Autodesk Inventor part; units mm, degrees
ref_plane "YZ Plane" through (0, 0, 0) normal (1, 0, 0) x (0, 1, 0)
ref_plane "XZ Plane" through (0, 0, 0) normal (0, 1, 0) x (-1, 0, 0)
ref_plane "XY Plane" through (0, 0, 0) normal (0, 0, 1) x (1, 0, 0)
sketch "Sketch1" plane through (0, 0, 0) normal (1, 0, 0) x (0, 1, 0)
  arc A0 (6.25, -17.1964) -> (-6.25, -17.1964) centre (0, -20) ccw
  line L0 (-6.25, -17.1964) -> (-6.25, -42.8036)
  line L1 (-6.25, -30) -> (6.25, -30) construction
  line L2 (0, 0) -> (0, -137.3205) construction
  arc A1 (-6.25, -42.8036) -> (6.25, -42.8036) centre (0, -40) ccw
  circle A2 centre (0, 0) radius 40 construction
  circle A3 centre (0, -20) radius 20 construction
  line L3 (6.25, -17.1964) -> (6.25, -42.8036)
  line L4 (0, 0) -> (17.3205, -10) construction
  line L5 (17.3205, -10) -> (34.641, -20) construction
  line L6 (-25, -137.3205) -> (25, -137.3205) construction
  line L7 (-18, -125.3205) -> (-18, -29)
  line L8 (22.5, -125.3205) -> (22.5, -100.3205)
  line L9 (-25, -120) -> (25, -120) construction
  line L10 (25, -120) -> (25, -137.3205) construction
  line L11 (-25, -120) -> (-25, -137.3205) construction
  line L12 (22.5, -109.2705) -> (17.5, -109.2705)
  line L13 (17.5, -109.2705) -> (17.5, -117.3705)
  line L14 (17.5, -117.3705) -> (22.5, -117.3705)
  line L15 (-15, -106.3205) -> (17.5, -106.3205) construction
  line L16 (17.5, -106.3205) -> (17.5, -149.3205) construction
  line L17 (17.5, -149.3205) -> (-15, -149.3205) construction
  line L18 (-15, -149.3205) -> (-15, -106.3205) construction
  line L19 (-15, -106.3205) -> (17.5, -149.3205) construction
  line L20 (17.5, -106.3205) -> (-15, -149.3205) construction
  line L21 (1.25, -106.3205) -> (1.25, -149.3205) construction
  line L22 (22.5, -109.3205) -> (17.5, -109.3205) construction
  line L23 (17.5, -117.3205) -> (22.5, -117.3205) construction
  line L24 (17.5, -113.3205) -> (22.5, -113.3205) construction
  line L25 (-18, -100.3205) -> (22.5, -100.3205) construction
  circle A4 centre (0, 0) radius 4 construction
  circle A5 centre (20, -103.3205) radius 1.75 construction
  line L26 (20, -103.3205) -> (20, -123.3205) construction
  circle A6 centre (20, -123.3205) radius 1.75 construction
  line L27 (-18, -109.2705) -> (-13, -109.2705)
  line L28 (-13, -109.2705) -> (-13, -117.3705)
  line L29 (-13, -117.3705) -> (-18, -117.3705)
  line L30 (-15.5, -103.3205) -> (-15.5, -123.3205) construction
  line L31 (-15.5, -103.3205) -> (20, -103.3205) construction
  line L32 (-15.5, -123.3205) -> (20, -123.3205) construction
  arc A7 (-4.4, -42.3749) -> (4.4, -42.3749) centre (0, -40) ccw construction
  arc A8 (4.4, -17.6251) -> (-4.4, -17.6251) centre (0, -20) ccw construction
  line L33 (-4.4, -17.6251) -> (-4.4, -42.3749) construction
  line L34 (4.4, -42.3749) -> (4.4, -17.6251) construction
  line L35 (-18, -29) -> (-18, -11)
  circle A9 centre (0, 0) radius 7 construction
  arc A10 (18, -11) -> (-18, -11) centre (0, -11) ccw
  line L36 (18, -11) -> (18, -92.5263)
  line L37 (18, -92.5263) -> (22.5, -100.3205)
  line L38 (-15, -42.8036) -> (-15, -97.3205)
  line L39 (-15, -97.3205) -> (15, -97.3205)
  line L40 (15, -42.8036) -> (15, -97.3205)
  line L41 (-10.5, -100.3205) -> (15, -100.3205)
  line L42 (15, -100.3205) -> (15, -122.3205)
  line L43 (15, -122.3205) -> (-10.5, -122.3205)
  line L44 (-10.5, -122.3205) -> (-10.5, -100.3205)
  line L45 (-15, -39.8036) -> (-9, -39.8036)
  arc A11 (-6.5383, 2.5) -> (-15, -11) centre (0, -11) ccw
  arc A12 (-6.5383, 2.5) -> (-1.5, -6.8374) centre (0, 0) ccw
  line L46 (-15, -11) -> (-15, -39.8036)
  line L47 (9, -39.8036) -> (9, -20)
  line L48 (15, -39.8036) -> (9, -39.8036)
  arc A13 (15, -11) -> (6.5383, 2.5) centre (0, -11) ccw
  arc A14 (1.5, -6.8374) -> (6.5383, 2.5) centre (0, 0) ccw
  line L49 (15, -11) -> (15, -39.8036)
  arc A15 (-8.5522, -42.8036) -> (8.5522, -42.8036) centre (0, -40) ccw
  line L50 (-15, -42.8036) -> (-8.5522, -42.8036)
  line L51 (-9, -39.8036) -> (-9, -20)
  arc A16 (-1.5, -11.1259) -> (-9, -20) centre (0, -20) ccw
  line L52 (-1.5, -6.8374) -> (-1.5, -11.1259)
  line L53 (15, -42.8036) -> (8.5522, -42.8036)
  arc A17 (9, -20) -> (1.5, -11.1259) centre (0, -20) ccw
  line L54 (1.5, -6.8374) -> (1.5, -11.1259)
  line L55 (-18, -137.3205) -> (-18, -100.3205) construction
  circle A18 centre (-15.5, -103.3205) radius 1.75 construction
  line L56 (22.5, -100.3205) -> (22.5, -137.3205) construction
  line L57 (-18, -125.3205) -> (22.5, -125.3205)
  arc A19 (19.6213, -109.2705) -> (17.5, -111.3918) centre (18.5607, -110.3312) ccw
  arc A20 (17.5, -115.2492) -> (19.6213, -117.3705) centre (18.5607, -116.3098) ccw
  arc A21 (-13, -111.3918) -> (-15.1213, -109.2705) centre (-14.0607, -110.3312) ccw
  arc A22 (-15.1213, -117.3705) -> (-13, -115.2492) centre (-14.0607, -116.3098) ccw
  line L58 (2.25, -122.3205) -> (2.25, -100.3205) construction
  point P0 (5.3819, -44.2376)
  point P1 (6.25, -41.5156)
  point P2 (17.5, -112.2705)
  point P3 (17.5, -114.3705)
  point P4 (1.25, -127.8205)
  point P5 (-13, -111.3918)
  point P6 (-13, -114.8191)
  point P7 (9, -20)
  point P8 (-13, -115.2492)
  point P9 (19.6213, -117.3705)
  point P10 (17.5, -115.2492)
  point P11 (17.5, -111.3918)
  dimension "d2" = 12.5
  dimension "d3" = 60
  dimension "d4" = 20
  dimension "d5" = 20
  dimension "d6" = 20
  dimension "d12" = 17.3205
  dimension "d13" = 120
  dimension "d17" = 32.5
  dimension "d18" = 43
  dimension "d19" = 9.5
  dimension "d21" = 0.05
  dimension "d24" = 3
  dimension "d25" = 9
  dimension "d26" = 6
  dimension "d36" = 8
  dimension "d48" = 50
  dimension "d50" = 3
  dimension "d51" = 3.5
  dimension "d56" = 8.8
  dimension "d57" = 5
  dimension "d58" = 1.85
  dimension "d59" = 1.85
  dimension "d65" = 14
  dimension "d66" = 30
  dimension "d70" = 3
  dimension "d74" = 3
  dimension "d81" = 7
  dimension "d82" = 5
  dimension "d85" = 5
  dimension "d86" = 2.5
  dimension "d91" = 8
  dimension "d92" = 8
  dimension "d93" = 3
  dimension "d95" = 3
  dimension "d96" = 3
  dimension "d97" = 9
  dimension "d99" = 1.5
extrude "Extrusion1" add sketch "Sketch1" along normal blind 3 contours L7 L29 A22 L28 A21 L27 L35 A10 L36 L37 L8 L12 A19 L13 A20 L14 L57
hole "Phi8.0-H7" at (0, 0, 0) direction (1, 0, 0) diameter 8 end through all
hole "Phi3.5" at (0, 20, -103.3205) at (0, -15.5, -103.3205) direction (1, 0, 0) diameter 3.5 end through all
fillet "R2" radius 2 25 edges at (1.5, -6.25, -17.1964) (1.5, -6.25, -42.8036) (1.5, 6.25, -42.8036) (1.5, 6.25, -17.1964) (1.5, 18, -92.5263) (1.5, -6.5383, 2.5) (1.5, -1.5, -6.8374) (1.5, 1.5, -6.8374) (1.5, 6.5383, 2.5) (1.5, -1.5, -11.1259) (1.5, 1.5, -11.1259) (1.5, -15, -39.8036) (1.5, -9, -39.8036) (1.5, 9, -39.8036) (1.5, 15, -39.8036) (1.5, 15, -97.3205) (1.5, -15, -97.3205) (1.5, -15, -42.8036) (1.5, -8.5522, -42.8036) (1.5, 8.5522, -42.8036) (1.5, 15, -42.8036) (1.5, 15, -122.3205) (1.5, 15, -100.3205) (1.5, -10.5, -100.3205) (1.5, -10.5, -122.3205)
chamfer "C0.5" distance 0.75 angle 45 6 edges at (1.5, 22.5, -109.2705) (1.5, 22.5, -117.3705) (1.5, -18, -117.3705) (1.5, -18, -109.2705) (1.5, -18, -125.3205) (1.5, 22.5, -125.3205)
equation "\"d6\" = d4"
properties part number "UpperArmFrame" material "CFRP"
Can you work these out from the model? Positions are in its coordinate system, mm. A direction names the side the tool comes from. Round coordinates to 2 decimals unless told otherwise and drop trailing zeros. Write each loop counter-clockwise with the first axis right and the second up, starting at its lowest first coordinate (ties: lowest second). Pieces come first, ordered by that corner, then holes. Notation, with made-up numbers: M 2.5,22 L 17.5,22 A21 cw 17.5,29 Z; hole C 34,-36.5 d8. An arc over 180 degrees is marked long. Use CSV: the item, a comma, the result in double quotes.
(1) We'd pull the mould along Z, two halves only. Please class faces 6 (the flat face through (1, 21, -117.37)), 7 (the flat face through (1, -18, -121)), 8 (the flat face through (1, 2, -125.32)): +Z half, -Z half, draft (parallel to the pull), parting line (faces both ways), or undercut.
Check values:
face 6,"undercut"
face 7,"draft"
face 8,"-Z half"
(2) Imagine slicing it at D-D (x = 0.75). Count the separate pieces of the cut face and the enclosed holes in it, plus the area to 3 significant figures.
Check values:
separate pieces,"1"
enclosed holes,"8"
area,"1,510 mm^2"
(3) Imagine slicing it at A-A (z = -113.5). Write out the boundary of the cut face in (x, y).
Check values:
outline,"M 0,-13 L 3,-13 L 3,-10.5 L 0,-10.5 Z; M 0,15 L 3,15 L 3,17.5 L 0,17.5 Z"
(4) Imagine slicing it at B-B (z = -15). Write out the boundary of the cut face in (x, y).
Check values:
outline,"M 0,-18 L 3,-18 L 3,-15 L 0,-15 Z; M 0,-7.48 L 3,-7.48 L 3,-4.68 L 0,-4.68 Z; M 0,4.68 L 3,4.68 L 3,7.48 L 0,7.48 Z; M 0,15 L 3,15 L 3,18 L 0,18 Z"
(5) I need wall thicknesses on line 1 along Y through (x, z) = (1, -23.5); line 2 along Y through (x, z) = (1.25, -103.5); line 3 along Y through (x, z) = (1.45, -51.5). Which ranges of each line are inside material? Lowest first, please.
Check values:
line 1,"-18 to -15, -9 to -6.25, 6.25 to 9, 15 to 18"
line 2,"-18 to -17.24, -13.76 to -10.5, 15 to 18.26, 21.74 to 22.5"
line 3,"-18 to -15, 15 to 18"
(6) I'm going to push flat-ended pins straight in: pin 1 (1.5 mm diameter, centred on x = 1.5, z = -79, fed in from +Y); pin 2 (8 mm diameter, centred on y = -1, z = -107, fed in from -X); pin 3 (1 mm diameter, centred on x = 2, z = -9, fed in from -Y); pin 4 (0.6 mm diameter, centred on x = 1.5, y = -12.5, fed in from +Z). Where does each tip first touch, or does it pass through?
Check values:
pin 1,"y = 18"
pin 2,"through"
pin 3,"y = -17.94"
pin 4,"z = 2.23"
(7) On a 3-axis mill with a long thin cutter (end or side, diameter ignored), from which of +Z, -Z, +X, -X, +Y, -Y can I reach the whole of each face in a straight line? I mean faces 1 (the flat face through (1, 18, -51)), 2 (the flat face through (1, -16, -117.37)), 3 (the flat face through (1, 22.5, -104)), 4 (the cylindrical face through (1.48, -5.46, -4.38)), 5 (the cylindrical face through (1, 0, 7)). Say none if no direction works.
Check values:
face 1,"+Z, +X, -X, +Y"
face 2,"+X, -X, -Y"
face 3,"+Z, -Z, +X, -X, +Y"
face 4,"+X, -X"
face 5,"+Z, +X, -X"
(8) Imagine slicing it at C-C (z = -53). Write out the boundary of the cut face in (x, y), plus the area to 3 significant figures.
Check values:
outline,"M 0,-18 L 3,-18 L 3,-15 L 0,-15 Z; M 0,15 L 3,15 L 3,18 L 0,18 Z"
area,"18.0 mm^2"
